Read the model definition and answer for the solid it produces. Units are mm, in the model's axes. Face numbers are marked on the shaded views. Give positions to 0.01 mm unless a question says otherwise; leave off trailing zeros. Write each loop counter-clockwise with the first axis right and the second up, starting at its lowest first coordinate (ties: lowest second). Pieces come first, ordered by that corner, then holes. Notation, with made-up numbers: M 76.25,72 L 101.25,72 A23 ccw 101.25,106 Z; hole C 85,46.25 d4. An arc over 180 degrees is marked long. Use a Markdown table: item, result. Add a question column.
Item 1: A cutting plane is placed at C-C on x = -21.5. Determine the outline of the cut face in (y, z).
Item 2: Given P1, Ø10, axis at x = 5.5, z = 22, coming from the +Y side, flat-ended and moving along its own axis, determine where the tip first touches the part or whether it passes through.
Item 3: A cutting plane is placed at B-B on y = 36.5. Determine the outline of the cut face in (x, z).
Item 4: A cutting plane is placed at A-A on z = 18.75. Determine the outline of the cut face in (x, y).
Item 5: Consider probe 1 along Z at (x, y) = (-12, -43.5); probe 2 along Y at (x, z) = (8, 22). Determine where each line is inside the solid, lowest interval first. Write a range as [from, to].
Item 6: The mould has two halves that part along X. Classify the marked faces 1, 2 and 3: pulls with the +X half, pulls with the -X half, needs draft (parallel to the pull), parting line crosses it, or undercut.
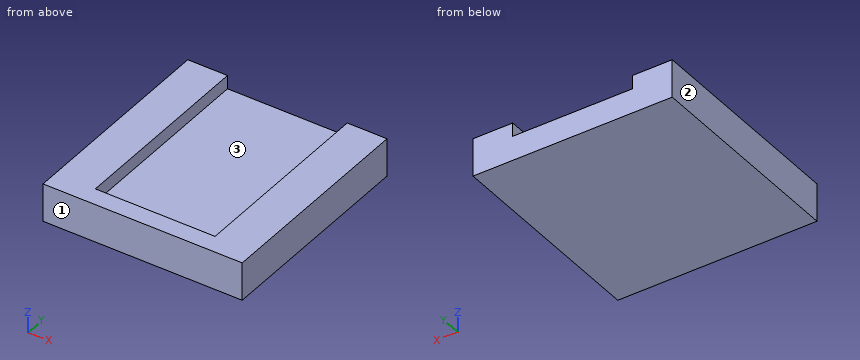
from build123d import *

# Parameters (mm, degrees)
F1_DEPTH  = 15
F1_FACE_W = 131
F1_FACE_H = 140
F2_DEPTH  = 10
F4_DEPTH  = 8.89


with BuildPart() as f1:
    # F0 (on Top) → F1 (new body)
    with BuildSketch(Plane.XY):
        Polygon((-65.5, 70), (-65.5, 0), (-65.5, -70), (0, -70), (65.5, -70), (65.5, -69.559447), (65.5, 0), (65.5, 70), (0, 70), align=None)
    extrude(amount=F1_DEPTH)

    # F1_face (on face) → F2 (join)
    with BuildSketch(Plane.XY.offset(15)):
        Rectangle(F1_FACE_W, F1_FACE_H)
    extrude(amount=F2_DEPTH)

    # F3 (on face) → F4 (cut)
    with BuildSketch(Plane.XY.offset(25)):
        Polygon((39.37, 70), (0, 70), (-39.37, 70), (-39.37, -57.848956), (0, -57.848956), (39.37, -57.848956), align=None)
    extrude(amount=-F4_DEPTH, mode=Mode.SUBTRACT)


solid = f1.part
Filled in:
| question | item | result |
|---|---|---|
| 1 | outline | M -70,0 L 70,0 L 70,16.11 L -57.85,16.11 L -57.85,25 L -70,25 Z |
| 2 | P1 | y = -57.85 |
| 3 | outline | M -65.5,0 L 65.5,0 L 65.5,25 L 39.37,25 L 39.37,16.11 L -39.37,16.11 L -39.37,25 L -65.5,25 Z |
| 4 | outline | M -65.5,-70 L 65.5,-70 L 65.5,70 L 39.37,70 L 39.37,-57.85 L -39.37,-57.85 L -39.37,70 L -65.5,70 Z |
| 5 | probe 1 | [0, 16.11] |
| 5 | probe 2 | [-70, -57.85] |
| 6 | face 1 | needs draft |
| 6 | face 2 | pulls with the -X half |
| 6 | face 3 | undercut |
